Read the model definition and answer for the solid it produces. Units are mm, in the model's axes. Face numbers are marked on the shaded views. A direction names the side the tool comes from. Round coordinates to 2 decimals unless told otherwise and drop trailing zeros. Order: outer loops, then holes, each group sorted by start corner. A loop starts at its lowest first (then second) coordinate and runs counter-clockwise, first axis right, second up. Notation, with made-up numbers: (46, 35.25) - (72, 35.25) arc R25 cw to (72, 48.25) - close; hole circle Ø6 at (19, 12). An arc over 180 degrees is marked (long way). Put each result on its own line as item: value. Start each with the question number.
Q1. Each of these flat-tipped pins is pushed along its axis until it touches: pin 1 Ø6 at (x, y) = (10, 2) entering from +Z; pin 2 Ø3 at (y, z) = (7, -9) entering from -X; pin 3 Ø1.5 at (y, z) = (10, 0.5) entering from +X; pin 4 Ø1 at (x, y) = (0, 7) entering from -Z. Where does it stop, or does it pass through?
Q2. Section D-D on z = 6.75 is taken. Give the vertices of the cut face in (x, y), then the cut area to 3 significant figures.
Q3. For a pull along Z with two mould halves and no side action, classify the marked faces 3, 4 and 5 as pulls with the +Z half, pulls with the -Z half, needs draft (parallel to the pull), parting line crosses it, or undercut.
Q4. Section C-C on y = 13 is taken. Give the vertices of the cut face in (x, z).
Q5. Section B-B on x = 5.5 is taken. Give the vertices of the cut face in (y, z), then the cut area to 3 significant figures.
Q6. Section A-A on z = 4 is taken. Give the vertices of the cut face in (x, y), then the cut area to 3 significant figures.
Q7. Which of the six approach directions +Z, -Z, +X, -X, +Y, -Y give full straight-line access (tool end or side, diameter ignored) to the marked faces 1 and 2?
Q8. Find the intervals of material crossed by line 1 along X through (y, z) = (4, -4); line 2 along Y through (x, z) = (-3, -9.75); line 3 along Z through (x, y) = (-6.25, 12.25), in increasing order. Write a range as from..to.
from build123d import *

# Parameters (mm, degrees)
SKETCH_2_R      = 12.5
EXTRUDE_1_DEPTH = 3
SKETCH_3_R      = 1.9
EXTRUDE_2_DEPTH = 11.5


with BuildPart() as part:
    # 草图2 → 凸台-拉伸1 (new body)
    with BuildSketch(Plane(origin=(0, 0, 0), x_dir=(1, 0, 0), z_dir=(0, 1, 0))):
        with Locations(Location((0, 0, 0), (0, 0, 270))):
            Circle(SKETCH_2_R)
    extrude(amount=EXTRUDE_1_DEPTH)

    # 草图3 → 凸台-拉伸2 (add)
    with BuildSketch(Plane(origin=(0, 3, 0), x_dir=(1, 0, 0), z_dir=(0, 1, 0))):
        with Locations(Location((0, 8, 0), (0, 0, 270))):
            Circle(SKETCH_3_R)
        with Locations(Location((6.92820323, 4, 0), (0, 0, 270))):
            Circle(SKETCH_3_R)
        with Locations(Location((6.92820323, -4, 0), (0, 0, 270))):
            Circle(SKETCH_3_R)
        with Locations(Location((0, -8, 0), (0, 0, 270))):
            Circle(SKETCH_3_R)
        with Locations(Location((-6.92820323, -4, 0), (0, 0, 270))):
            Circle(SKETCH_3_R)
        with Locations(Location((-6.92820323, 4, 0), (0, 0, 270))):
            Circle(SKETCH_3_R)
    extrude(amount=EXTRUDE_2_DEPTH)


solid = part.part
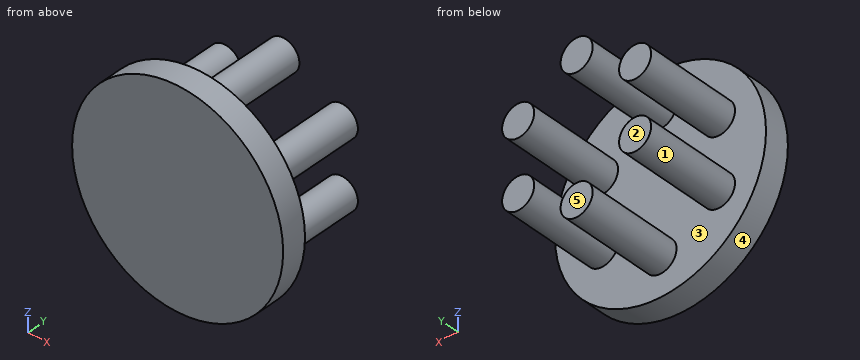
Findings:
1. pin 1: z = 10.36
1. pin 2: x = -1.9
1. pin 3: through
1. pin 4: z = -9.9
2. outline: (-10.52, 0) - (10.52, 0) - (10.52, 3) - (1.43, 3) - (1.43, 14.5) - (-1.43, 14.5) - (-1.43, 3) - (-10.52, 3) - close
2. area: 96.0 mm2
3. face 3: undercut
3. face 4: parting line crosses it
3. face 5: needs draft
4. outline: circle Ø3.8 at (-6.93, -4); circle Ø3.8 at (-6.93, 4); circle Ø3.8 at (0, -8); circle Ø3.8 at (0, 8); circle Ø3.8 at (6.93, -4); circle Ø3.8 at (6.93, 4)
5. outline: (0, -11.22) - (3, -11.22) - (3, -5.25) - (14.5, -5.25) - (14.5, -2.75) - (3, -2.75) - (3, 2.75) - (14.5, 2.75) - (14.5, 5.25) - (3, 5.25) - (3, 11.22) - (0, 11.22) - close
5. area: 125 mm2
6. outline: (-11.84, 0) - (11.84, 0) - (11.84, 3) - (8.83, 3) - (8.83, 14.5) - (5.03, 14.5) - (5.03, 3) - (-5.03, 3) - (-5.03, 14.5) - (-8.83, 14.5) - (-8.83, 3) - (-11.84, 3) - close
6. area: 158 mm2
7. face 1: +Y
7. face 2: +Z, -Z, +X, -X, +Y
8. line 1: -8.83..-5.03, 5.03..8.83
8. line 2: 0..3
8. line 3: -5.77..-2.23, 2.23..5.77
